For this review, take the finished solid that the model builds, in its own axes (mm). A direction names the side the tool comes from. Round coordinates to 2 decimals unless told otherwise and drop trailing zeros. Loops run counter-clockwise (first coordinate to the right, second up) from the corner with the lowest first, then second, coordinate; pieces in that order, holes last. Notation, with made-up numbers: M -24,31.5 L 14,31.5 A24 cw 14,68.5 Z; hole C -17.5,73 d4. An arc over 180 degrees is marked long. One line per question, with ' | ' between items. Start each with the question number.
1) For probe 1 along Y at (x, z) = (0, -1.95); probe 2 along X at (y, z) = (0, -24.6), list the stretches that pass through material, from the lowest coordinate up. Write a range as from..to.
2) We need section B-B (y = 1.5). State how many separate pieces and enclosed holes the cut face has, and give its area (3 significant figures).
3) For faces 4 (the face through (-10, -3.2, -2.7)), 5 (the face through (-2, 5, -20.7)), 6 (the face through (-2.5, 0, -19)), 7 (the face through (-12.932, 5.362, -2.958)), 8 (the face through (-2.2, -0.1, -26.7)), list the 3-axis set-ups (+Z, -Z, +X, -X, +Y, -Y) from which the entire face can be reached by the end or side of a thin tool; tool diameter is ignored.
4) Mouldability with a two-part tool opening along X and no side actions: class faces 1 (the face through (1.89, 8.53, -14.79)), 2 (the face through (-9.3, 9.3, 0)), 3 (the face through (10.316, -7.91, -3.042)) as pulls with the +X half, pulls with the -X half, needs draft (parallel to the pull), parting line crosses it, or undercut.
5) We need section A-A (z = -12). Give the boundary of the cut face in (x, y), and give its area (3 significant figures).
6) For pin 1 Ø1 at (x, z) = (1, -2) entering from +Y; pin 2 Ø4.5 at (y, z) = (-1, -18) entering from +X; pin 3 Ø4.5 at (y, z) = (0, -18.6) entering from +X; pin 4 Ø2.5 at (x, y) = (0, 0) entering from -Z, all flat-tipped, find the tip position at first contact; note any pin that passes through.
7) We need section C-C (z = -8). Give the boundary of the cut face in (x, y).
Autodesk Inventor part; units mm, degrees
ref_plane "YZ Plane" through (0, 0, 0) normal (1, 0, 0) x (0, 1, 0)
ref_plane "XZ Plane" through (0, 0, 0) normal (0, 1, 0) x (-1, 0, 0)
ref_plane "XY Plane" through (0, 0, 0) normal (0, 0, 1) x (1, 0, 0)
sketch "Sketch1" plane through (0, 0, 0) normal (0, 1, 0) x (-1, 0, 0)
  line L0 (0, -27.5114) -> (0, 22.3977)
  line L1 (11.5, -6) -> (10.5, -6)
  line L2 (10.5, -6) -> (10.5, 0)
  line L3 (10.5, 0) -> (11.5, 0)
  line L4 (11.5, 0) -> (11.5, -6)
  line L5 (14, -7.5) -> (10.5, -7.5)
  line L6 (10.5, -5.5121) -> (10.5, -6)
  line L7 (10.5, -6) -> (14, -6)
  line L8 (14, -6) -> (14, -5.8832)
  line L9 (28.1307, 0) -> (-27.0173, 0)
  line L10 (7.5, -25.7) -> (6.5, -25.7)
  line L11 (6.5, -25.7) -> (6.5, -20.7)
  line L12 (6.5, -20.7) -> (7.5, -20.7)
  line L13 (7.5, -20.7) -> (7.5, -25.7)
  line L14 (5, -26.7) -> (2, -26.7)
  line L15 (2, -26.7) -> (2, -20.7)
  line L16 (2, -20.7) -> (5, -20.7)
  line L17 (5, -20.7) -> (5, -26.7)
  line L18 (7.5, -20.7) -> (2, -20.7)
  line L19 (2, -20.7) -> (2, -18.4879)
  line L20 (2, -16.5) -> (7.5, -16.5)
  line L21 (7.5, -18.1168) -> (7.5, -20.7)
  line L22 (3.3649, -15.0548) -> (9.1351, -8.9452)
  line L23 (8.4466, -15.1893) -> (13.0534, -8.8107)
  arc A0 (8.4466, -15.1893) -> (7.5, -18.1168) centre (12.5, -18.1168) ccw
  arc A1 (13.0534, -8.8107) -> (14, -5.8832) centre (9, -5.8832) ccw
  arc A2 (9.1351, -8.9452) -> (10.5, -5.5121) centre (5.5, -5.5121) ccw
  arc A3 (3.3649, -15.0548) -> (2, -18.4879) centre (7, -18.4879) ccw
  line L24 (13, -6) -> (14, -6)
  line L25 (14, -6) -> (14, 0)
  line L26 (14, 0) -> (13, 0)
  line L27 (13, 0) -> (13, -6)
  line L28 (11.5, 0) -> (11.5, 6)
  line L29 (11.5, 6) -> (11.4, 6)
  line L30 (11.4, 6) -> (10.5, 0)
  point P0 (0, 0)
  point P1 (11.5, -6)
  point P2 (13.9986, -6)
  point P3 (10.5, -5.5121)
  dimension "d2" = 1
  dimension "d4" = 1.5
  dimension "d5" = 6
  dimension "d6" = 6.5
  dimension "d7" = 1.5
  dimension "d8" = 1
  dimension "d9" = 4.2
  dimension "d10" = 5
  dimension "d11" = 9
  dimension "d12" = 2
  dimension "d13" = 5
  dimension "d14" = 5
  dimension "d15" = 5
  dimension "d17" = 6
  dimension "d20" = 1
  dimension "d21" = 6
  dimension "d22" = 1.5
  dimension "d23" = 13
  dimension "d28" = 6
  dimension "d29" = 0.1
revolve "Revolution1" add sketch "Sketch1" angle 360 about axis through (0, 0, -27.5114) along (0, 0, 1) contours L7 A1 L23 A0 L21 L12 L18 L16 L19 A3 L22 A2 L2 L1 | L1 L2 L3 L4 | L3 L30 L29 L28 | L27 L9 L25 L8 L7 | L16 L17 L14 L15 | L13 L10 L11 L12
sketch "Sketch2" plane through (0, 0, 0) normal (1, 0, 0) x (0, 1, 0)
  line L0 (5, -26.7) -> (-5, -26.7) construction
  line L1 (0, -26.7) -> (0, -18.4879)
  line L2 (2, -18.4879) -> (-2, -18.4879) construction
  line L3 (5, -20.7) -> (-5, -20.7) construction
  circle A0 centre (0, -18.6) radius 2
  point P0 (0, 0)
  dimension "d18" = 4
  dimension "d19" = 2.1
extrude "Extrusion1" cut sketch "Sketch2" along normal blind 14 and the other way blind 2.5
equation "\"d18\" = ft_D"
equation "\"d19\" = 0.5 * ft_D + tol"
equation "\"d24\" = sv_OD + hw_thickness"
equation "\"d26\" = 0.5 * hw_thickness + 0.5 * ft_D"
equation "\"d2\" = hw_thickness"
equation "\"d4\" = 0.25 * hw_length"
equation "\"d5\" = hw_length"
equation "\"d7\" = sv_thickness"
equation "\"d8\" = hw_thickness"
equation "\"d9\" = 1.05 * ft_D"
equation "\"d10\" = 0.833333 * hw_length"
equation "\"d11\" = 1.5 * hw_length"
equation "\"d13\" = fillet_D"
equation "\"d14\" = fillet_D"
equation "\"d15\" = fillet_D"
equation "\"d17\" = hw_length"
equation "\"d20\" = hw_thickness"
equation "\"d21\" = hw_length"
equation "\"d22\" = lv_thickness"
equation "\"d28\" = hw_length"
equation "\"d29\" = tol"
equation "\"lv_OD\" = 26"
equation "\"lv_thickness\" = 1.5"
equation "\"hw_thickness\" = 1"
equation "\"hw_length\" = 6"
equation "\"sv_OD\" = 13"
equation "\"sv_thickness\" = 1.5"
equation "\"ft_D\" = 4"
equation "\"fillet_D\" = 5"
equation "\"tol\" = 0.1"
properties part number "fly_funnel"
Answers below:
1) probe 1: -14..-13, -11.5..-10.5, 10.5..11.5, 13..14 | probe 2: -7.5..-6.5, -5..-2, 2..5, 6.5..7.5
2) separate pieces: 3 | enclosed holes: 0 | area: 208 mm^2
3) face 4: +Z | face 5: -Z | face 6: +X | face 7: +Z, -Z | face 8: -Z, +X, -X, +Y, -Y
4) face 1: parting line crosses it | face 2: needs draft | face 3: undercut
5) outline: C 0,0 d21.5; hole C 0,0 d12.5 | area: 240 mm^2
6) pin 1: y = 13.99 | pin 2: x = 8.05 | pin 3: x = 7.82 | pin 4: through
7) outline: C 0,0 d27.06; hole C 0,0 d19.67
